The listing builds one solid part. Answer for the finished solid, in the listing's coordinates (mm). A direction names the side the tool comes from. Give positions to 0.01 mm unless a question says otherwise; leave off trailing zeros. Order: outer loops, then holes, each group sorted by start corner. A loop starts at its lowest first (then second) coordinate and runs counter-clockwise, first axis right, second up. Notation, with made-up numbers: (-35.75, 69.25) - (16.25, 69.25) arc R19 ccw to (16.25, 98.25) - close; hole circle Ø5 at (85, 3.25). An arc over 180 degrees is marked (long way). Use CSV: the item, a comma, the result in double quotes.
```python
from build123d import *

# Parameters (mm, degrees)
SKETCH1_W                    = 20
SKETCH1_H                    = 55
BASE_FLANGE1_DEPTH           = 0.7
EDGE_FLANGE1_STRIP_CUT_DEPTH = 20
EDGE_FLANGE1_DEPTH           = 20
EDGE_FLANGE2_STRIP_CUT_DEPTH = 20
EDGE_FLANGE2_DEPTH           = 20
F_19_0_166_DIAMETER_SLOT1_D  = 4.2164
F_19_0_166_DIAMETER_SLOT2_D  = 4.2164


# Sheet-metal steps are written as plain solids
with BuildPart() as part:
    # Sketch1 → Base-Flange1 (new body)
    with BuildSketch(Plane.XY):
        Rectangle(SKETCH1_W, SKETCH1_H)
    extrude(amount=-BASE_FLANGE1_DEPTH)

    # Edge-Flange1 strip (across the edge) → Edge-Flange1 strip cut (cut)
    with BuildSketch(Plane(origin=(-10, -27.5, 0), x_dir=(0, 0.7071067811865438, 0.7071067811865512), z_dir=(1, 0, 0))):
        Polygon((-3.371930009, 2.381980515), (-0.260660172, -0.729289322), (0.234314575, -0.234314575), (-2.876955262, 2.876955262), align=None)
    extrude(amount=EDGE_FLANGE1_STRIP_CUT_DEPTH, mode=Mode.SUBTRACT)

    # Edge-Flange1 section (across the edge) → Edge-Flange1 (add)
    with BuildSketch(Plane(origin=(-10, -27.5, 0), x_dir=(0, 0.7071067811865438, 0.7071067811865512), z_dir=(1, 0, 0))):
        with BuildLine():
            Line((-0.7, 0.33137085), (-0.7, 10))
            Line((-0.7, 10), (0, 10))
            Line((0, 10), (0, 0.33137085))
            ThreePointArc((0, 0.33137085), (0.060896374, 0.025224104), (0.234314575, -0.234314575))
            Line((0.234314575, -0.234314575), (-0.260660172, -0.729289322))
            ThreePointArc((-0.260660172, -0.729289322), (-0.585819299, -0.242654299), (-0.7, 0.33137085))
        make_face()
    extrude(amount=EDGE_FLANGE1_DEPTH)

    # Edge-Flange2 strip (across the edge) → Edge-Flange2 strip cut (cut)
    with BuildSketch(Plane(origin=(10, 27.5, 0), x_dir=(0, -0.7071067811865438, 0.7071067811865512), z_dir=(-1, 0, 0))):
        Polygon((-3.371930009, 2.381980515), (-0.260660172, -0.729289322), (0.234314575, -0.234314575), (-2.876955262, 2.876955262), align=None)
    extrude(amount=EDGE_FLANGE2_STRIP_CUT_DEPTH, mode=Mode.SUBTRACT)

    # Edge-Flange2 section (across the edge) → Edge-Flange2 (add)
    with BuildSketch(Plane(origin=(10, 27.5, 0), x_dir=(0, -0.7071067811865438, 0.7071067811865512), z_dir=(-1, 0, 0))):
        with BuildLine():
            Line((-0.7, 0.33137085), (-0.7, 10))
            Line((-0.7, 10), (0, 10))
            Line((0, 10), (0, 0.33137085))
            ThreePointArc((0, 0.33137085), (0.060896374, 0.025224104), (0.234314575, -0.234314575))
            Line((0.234314575, -0.234314575), (-0.260660172, -0.729289322))
            ThreePointArc((-0.260660172, -0.729289322), (-0.585819299, -0.242654299), (-0.7, 0.33137085))
        make_face()
    extrude(amount=EDGE_FLANGE2_DEPTH)

    # #19 (0.166) Diameter Slot1 (through all)
    with Locations(Plane(origin=(0, -13.75, -13.75), x_dir=(1, 0, 0), z_dir=(0, 0.7071067811865438, 0.7071067811865513))):
        with Locations((0, -24.738773453)):
            Hole(F_19_0_166_DIAMETER_SLOT1_D / 2)

    # #19 (0.166) Diameter Slot2 (through all)
    with Locations(Plane(origin=(0, 13.75, -13.75), x_dir=(1, 0, 0), z_dir=(0, -0.7071067811865441, 0.7071067811865509))):
        with Locations((0, 24.940163898)):
            Hole(F_19_0_166_DIAMETER_SLOT2_D / 2)


solid = part.part
```
Item 1: The part is cut by section A-A (x = 7.75). Give the vertices of the cut face in (y, z), and give its area (3 significant figures).
Taken from the geometry:
outline,"(-35.07, 6.58) - (-28.23, -0.26) arc R1.5 ccw to (-27.17, -0.7) - (27.17, -0.7) arc R1.5 ccw to (28.23, -0.26) - (35.07, 6.58) - (34.57, 7.07) - (27.73, 0.23) arc R0.8 cw to (27.17, 0) - (-27.17, 0) arc R0.8 cw to (-27.73, 0.23) - (-34.57, 7.07) - close"
area,"52.8 mm^2"
Item 2: Which of the six approach directions +Z, -Z, +X, -X, +Y, -Y give full straight-line access (tool end or side, diameter ignored) to faces 3 (the face through (0.1, 29.7, 2.2)), 4 (the face through (0.274, 33.114, 5.112))?
Taken from the geometry:
face 3,"+Z, +X, -X"
face 4,"none"
Item 3: Each of these flat-tipped pins is pushed along its axis until it touches: pin 1 (3 mm diameter, centred on x = 7, y = 9, fed in from +Z); pin 2 (4 mm diameter, centred on x = -6.5, z = 3, fed in from +Y). Where does it stop, or does it pass through?
Taken from the geometry:
pin 1,"z = 0"
pin 2,"y = 33.49"
Item 4: The mould has two halves that part along X. Classify faces 1 (the face through (-2.4, -31.2, 3.7)), 2 (the face through (0.27, -30.02, 2.01)): +X half, -X half, draft (parallel to the pull), parting line (faces both ways), or undercut.
Taken from the geometry:
face 1,"draft"
face 2,"undercut"
Item 5: The part is cut by section B-B (y = 21). Give the vertices of the cut face in (x, z).
Taken from the geometry:
outline,"(-10, -0.7) - (10, -0.7) - (10, 0) - (-10, 0) - close"
Item 6: Find the intervals of material crossed by line 1 along Y through (x, z) = (-6.5, 2.5); line 2 along Y through (x, z) = (-4, 6.25); line 3 along Z through (x, y) = (6, 11.5), in increasing order.
Taken from the geometry:
line 1,"-30.99 to -30, 30 to 30.99"
line 2,"-34.74 to -33.75, 33.75 to 34.74"
line 3,"-0.7 to 0"
